from build123d import *

# Parameters (mm, degrees)
CROQUIS1_R              = 1.5
SALIENTE_EXTRUIR1_DEPTH = 3


with BuildPart() as part:
    # Croquis1 → Saliente-Extruir1 (new body)
    with BuildSketch(Plane.XY):
        with BuildLine():
            Line((0, -4), (-48, -4))
            Line((-48, -4), (-48, -7))
            Line((-48, -7), (12, -7))
            Line((12, -7), (12, 0))
            ThreePointArc((12, 0), (10.828427125, 2.828427125), (8, 4))
            Line((8, 4), (0, 4))
            ThreePointArc((0, 4), (-4, 0), (0, -4))
        make_face()
        Circle(CROQUIS1_R, mode=Mode.SUBTRACT)
        with Locations((8, 0)):
            Circle(CROQUIS1_R, mode=Mode.SUBTRACT)
    extrude(amount=SALIENTE_EXTRUIR1_DEPTH)


solid = part.part
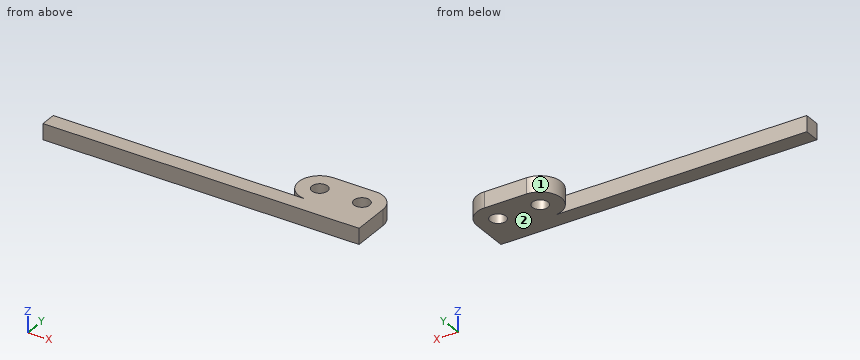
Model file for the job. Use its own axes, mm. Face numbers are marked on the shaded views. Coordinates: 2 decimals unless noted, no trailing zeros. Order: outer loops, then holes, each group sorted by start corner. A loop starts at its lowest first (then second) coordinate and runs counter-clockwise, first axis right, second up. Notation, with made-up numbers: (70, 7) -> (83, 7) arc R25 ccw to (83, 21) -> close; hole circle Ø8 at (54, -19.5). An arc over 180 degrees is marked (long way). Return JSON: item names as keys, results as strings. Group by question number.
Item 1: Wall check: line 1 along Y through (x, z) = (8, 1.2); line 2 along X through (y, z) = (0.5, 1.25); line 3 along Y through (x, z) = (-14, 0.95). Give the ranges that are in metal, low to high. Write a range as [from, to].
Item 2: Saw through at B-B on x = -2.5. Write the cut outline in (y, z), then the cut area to 3 significant figures.
Item 3: Saw through at A-A on z = 2.5. Write the cut outline in (x, y).
Item 4: Saw through at D-D on x = -29. Write the cut outline in (y, z), then the cut area to 3 significant figures.
Item 5: Saw through at C-C on y = 1. Write the cut outline in (x, z).
Item 6: Flat gauge pins, fed straight in: P1, Ø1.8, axis at x = 0, y = 0, coming from the +Z side; P2, Ø1, axis at x = -35.5, z = 2, coming from the +Y side. Where does each tip first touch, or does it go through?
Item 7: Pull direction Y, two halves, no side cores. Call the marked faces 1 and 2: pulls with the +Y half, pulls with the -Y half, needs draft (parallel to the pull), parting line crosses it, or undercut.
Values found:
{
 "1": {"line 1": "y = [-7, -1.5], [1.5, 4]", "line 2": "x = [-3.97, -1.41], [1.41, 6.59], [9.41, 11.97]", "line 3": "y = [-7, -4]"},
 "2": {"outline": "(-7, 0) -> (-4, 0) -> (-4, 3) -> (-7, 3) -> close; (-3.12, 0) -> (3.12, 0) -> (3.12, 3) -> (-3.12, 3) -> close", "area": "27.7 mm2"},
 "3": {"outline": "(-48, -7) -> (12, -7) -> (12, 0) arc R4 ccw to (8, 4) -> (0, 4) arc R4 ccw to (0, -4) -> (-48, -4) -> close; hole circle Ø3 at (0, 0); hole circle Ø3 at (8, 0)"},
 "4": {"outline": "(-7, 0) -> (-4, 0) -> (-4, 3) -> (-7, 3) -> close", "area": "9.00 mm2"},
 "5": {"outline": "(-3.87, 0) -> (-1.12, 0) -> (-1.12, 3) -> (-3.87, 3) -> close; (1.12, 0) -> (6.88, 0) -> (6.88, 3) -> (1.12, 3) -> close; (9.12, 0) -> (11.87, 0) -> (11.87, 3) -> (9.12, 3) -> close"},
 "6": {"P1": "passes through", "P2": "stops at y = -4"},
 "7": {"face 1": "undercut", "face 2": "needs draft"}
}
